```python
from build123d import *

# Parameters (mm, degrees)
SKETCH1_W             = 36
SKETCH1_H             = 10
BOSS_EXTRUDE1_DEPTH   = 12
SKETCH2_W             = 14
SKETCH2_H             = 12
BOSS_EXTRUDE2_DEPTH   = 19
SKETCH3_R             = 2.25
CUT_EXTRUDE1_DEPTH    = 11
SKETCH4_R             = 4
CUT_EXTRUDE2_DEPTH    = 4
M8_TAPPED_HOLE1_D     = 6.8
M8_TAPPED_HOLE1_DEPTH = 19.75
M8_TAPPED_HOLE1_TIP   = 2.042926105


with BuildPart() as part:
    # Sketch1 → Boss-Extrude1 (new body)
    with BuildSketch(Plane.XY):
        with Locations((9.722605043, -1.956268222)):
            Rectangle(SKETCH1_W, SKETCH1_H)
    extrude(amount=BOSS_EXTRUDE1_DEPTH)

    # Sketch2 → Boss-Extrude2 (add)
    with BuildSketch(Plane(origin=(0, 3.043731778, 0), x_dir=(1, 0, 0), z_dir=(0, 1, 0))):
        with Locations((20.722605043, -6)):
            Rectangle(SKETCH2_W, SKETCH2_H)
    extrude(amount=BOSS_EXTRUDE2_DEPTH)

    # Sketch3 → Cut-Extrude1 (cut, through all)
    with BuildSketch(Plane(origin=(0, 3.043731778, 0), x_dir=(1, 0, 0), z_dir=(0, 1, 0))):
        with Locations((-3.277394957, -6)):
            Circle(SKETCH3_R)
        with Locations((8.722605043, -6)):
            Circle(SKETCH3_R)
    extrude(amount=-CUT_EXTRUDE1_DEPTH, mode=Mode.SUBTRACT)

    # Sketch4 → Cut-Extrude2 (cut)
    with BuildSketch(Plane(origin=(0, 3.043731778, 0), x_dir=(1, 0, 0), z_dir=(0, 1, 0))):
        with Locations((-3.277394957, -6)):
            Circle(SKETCH4_R)
        with Locations((8.722605043, -6)):
            Circle(SKETCH4_R)
    extrude(amount=-CUT_EXTRUDE2_DEPTH, mode=Mode.SUBTRACT)

    # M8 Tapped Hole1
    with Locations(Plane(origin=(27.722605043, 0, 0), x_dir=(0, 0, -1), z_dir=(1, 0, 0))):
        with Locations((-6, 16.043731778)):
            Hole(M8_TAPPED_HOLE1_D / 2, depth=M8_TAPPED_HOLE1_DEPTH)
            with Locations((0, 0, -(M8_TAPPED_HOLE1_DEPTH + M8_TAPPED_HOLE1_TIP / 2))):  # 118° drill point
                Cone(0, M8_TAPPED_HOLE1_D / 2, M8_TAPPED_HOLE1_TIP, mode=Mode.SUBTRACT)


solid = part.part
```
Geometry: final body of the model. Coordinates: model frame, mm. A direction names the side the tool comes from. Round coordinates to 2 decimals unless told otherwise and drop trailing zeros. Write each loop counter-clockwise with the first axis right and the second up, starting at its lowest first coordinate (ties: lowest second). Pieces come first, ordered by that corner, then holes. Notation, with made-up numbers: (79.25, 42.25) -> (93.25, 42.25) arc R22 cw to (93.25, 52.25) -> close; hole circle Ø8 at (-37.75, -6.5). An arc over 180 degrees is marked (long way). Return JSON: item names as keys, results as strings.
Q1. Mould query, pull axis Z, two halves, no side actions, for faces 1 (the flat face through (13, 1, 12)), 2 (the cylindrical face through (10.869, -3.914, 5.324)), 3 (the flat face through (21, 22.044, 6)). Classes: +Z half, -Z half, draft (parallel to the pull), parting line (faces both ways), or undercut.
From the geometry:
{"face 1": "+Z half", "face 2": "undercut", "face 3": "draft"}
Q2. Ray query, line 1 (Z direction, x = 9, y = 0); line 2 (X direction, y = -4, z = 6); line 3 (X direction, y = -0.1, z = 6). Return the intervals inside material, ascending.
From the geometry:
{"line 1": "0 to 2.01, 9.99 to 12", "line 2": "-8.28 to -5.53, -1.03 to 6.47, 10.97 to 27.72", "line 3": "-8.28 to -7.28, 0.72 to 4.72, 12.72 to 27.72"}
Q3. Set-up query: faces 4 (the flat face through (3, 3.044, 6)), 5 (the cylindrical face through (-4.145, 1.072, 9.905)), 6 (the cylindrical face through (20.625, 17.065, 9.243)). Return all of +Z, -Z, +X, -X, +Y, -Y with unobstructed straight access to the full face (end or side cutting, diameter ignored); none if empty.
From the geometry:
{"face 4": "+Z, -Z, -X, +Y", "face 5": "+Y", "face 6": "+X, -X"}
Q4. Section C-C on y = -0.5. Return the cut outline in (x, z), and give its area (3 significant figures).
From the geometry:
{"outline": "(-8.28, 0) -> (27.72, 0) -> (27.72, 12) -> (-8.28, 12) -> close; hole circle Ø8 at (-3.28, 6); hole circle Ø8 at (8.72, 6)", "area": "331 mm2"}
Q5. First-contact query: pin 1 Ø6 at (x, z) = (8.72, 6) entering from +Y; pin 2 Ø6.5 at (x, z) = (10, 7) entering from +Y; pin 3 Ø1 at (y, z) = (8.5, 8.5) entering from -X. Flat tips, straight axial feed; report the tip coordinate or a pass-through.
From the geometry:
{"pin 1": "y = -0.96", "pin 2": "y = 3.04", "pin 3": "x = 13.72"}
Q6. Section A-A on z = 6. Return the cut outline in (x, y).
From the geometry:
{"outline": "(-8.28, -6.96) -> (-5.53, -6.96) -> (-5.53, -0.96) -> (-7.28, -0.96) -> (-7.28, 3.04) -> (-8.28, 3.04) -> close; (-1.03, -6.96) -> (6.47, -6.96) -> (6.47, -0.96) -> (4.72, -0.96) -> (4.72, 3.04) -> (0.72, 3.04) -> (0.72, -0.96) -> (-1.03, -0.96) -> close; (10.97, -6.96) -> (27.72, -6.96) -> (27.72, 12.64) -> (13.72, 12.64) -> (13.72, 3.04) -> (12.72, 3.04) -> (12.72, -0.96) -> (10.97, -0.96) -> close; (13.72, 19.44) -> (27.72, 19.44) -> (27.72, 22.04) -> (13.72, 22.04) -> close"}
Q7. Section B-B on x = -2. Return the cut outline in (y, z).
From the geometry:
{"outline": "(-6.96, 0) -> (3.04, 0) -> (3.04, 2.21) -> (-0.96, 2.21) -> (-0.96, 4.15) -> (-6.96, 4.15) -> close; (-6.96, 7.85) -> (-0.96, 7.85) -> (-0.96, 9.79) -> (3.04, 9.79) -> (3.04, 12) -> (-6.96, 12) -> close"}
Q8. Section D-D on x = 23. Return the cut outline in (y, z), and give its area (3 significant figures).
From the geometry:
{"outline": "(-6.96, 0) -> (22.04, 0) -> (22.04, 12) -> (-6.96, 12) -> close; hole circle Ø6.8 at (16.04, 6)", "area": "312 mm2"}
